Input: part model. Units: mm. Frame: model coordinates. A direction names the side the tool comes from. Round coordinates to 2 decimals unless told otherwise and drop trailing zeros. Write each loop counter-clockwise with the first axis right and the second up, starting at its lowest first coordinate (ties: lowest second). Pieces come first, ordered by that corner, then holes. Notation, with made-up numbers: (40.25, 44.25) - (46.25, 44.25) arc R6 ccw to (46.25, 52.25) - close; hole circle Ø7 at (66, 40.5). An arc over 180 degrees is marked (long way). Use one line per item in the form item = value.
```python
from build123d import *

# Parameters (mm, degrees)
F0_R     = 30.5
F1_DEPTH = 12
F0_R_2   = 5.5
F2_DEPTH = 3


with BuildPart() as f1:
    # F0 (on Top) → F1 (new body)
    with BuildSketch(Plane.XY):
        with Locations((-0.117735, 0.149164)):
            Circle(F0_R)
        with BuildLine():
            ThreePointArc((-18.165188, 22.593082), (-17.375002, 23.206196), (-16.564005, 23.791503))
            ThreePointArc((-16.564005, 23.791503), (22.939297, 17.406431), (17.929717, -22.294755))
            ThreePointArc((17.929717, -22.294755), (17.139532, -22.907869), (16.328534, -23.493176))
            ThreePointArc((16.328534, -23.493176), (-23.174768, -17.108103), (-18.165188, 22.593082))
        make_face(mode=Mode.SUBTRACT)
    extrude(amount=F1_DEPTH)

    # F0 (on Top) → F2 (join)
    with BuildSketch(Plane.XY):
        with BuildLine():
            Line((-3.165644, 5.890266), (-16.564005, 23.791503))
            ThreePointArc((-16.564005, 23.791503), (-17.375002, 23.206196), (-18.165188, 22.593082))
            Line((-18.165188, 22.593082), (-4.766827, 4.691844))
            ThreePointArc((-4.766827, 4.691844), (-5.321579, -3.745706), (2.930173, -5.591938))
            Line((2.930173, -5.591938), (16.328534, -23.493176))
            ThreePointArc((16.328534, -23.493176), (17.139532, -22.907869), (17.929717, -22.294755))
            Line((17.929717, -22.294755), (4.531356, -4.393517))
            ThreePointArc((4.531356, -4.393517), (5.086109, 4.044033), (-3.165644, 5.890266))
        make_face()
        with Locations((-0.117735, 0.149164)):
            Circle(F0_R_2, mode=Mode.SUBTRACT)
    extrude(amount=F2_DEPTH)


solid = f1.part
```
(1) Cut plane C-C on x = 22. Output: boundary loops of the cut face in (y, z).
Derived:
outline = (-20.85, 0) - (-18.3, 0) - (-18.3, 12) - (-20.85, 12) - close; (18.59, 0) - (21.15, 0) - (21.15, 12) - (18.59, 12) - close
(2) Draft query along X for faces 1 (the face through (5.16, 3.94, 1.48)), 2 (the face through (16.279, 25.867, 5.916)), 3 (the face through (9.54, -14.42, 1.48)), 4 (the face through (11, -27, 12)). Return one class per face: released by +X, released by -X, zero draft, split by the parting line, or undercut.
Derived:
face_1 = undercut
face_2 = split by the parting line
face_3 = undercut
face_4 = zero draft
(3) First-contact query: pin 1 Ø4 at (y, z) = (19, 10.5) entering from -X; pin 2 Ø1.5 at (y, z) = (-9, 2) entering from -X; pin 3 Ø5 at (x, z) = (1.5, 1.5) entering from +Y. Flat tips, straight axial feed; report the tip coordinate or a pass-through.
Derived:
pin_1 = -25.54
pin_2 = -29.44
pin_3 = 30.65
(4) Cut plane A-A on x = -8. Output: boundary loops of the cut face in (y, z).
Derived:
outline = (-29.31, 0) - (-27.55, 0) - (-27.55, 12) - (-29.31, 12) - close; (9.01, 0) - (12.35, 0) - (12.35, 3) - (9.01, 3) - close; (27.85, 0) - (29.61, 0) - (29.61, 12) - (27.85, 12) - close
(5) Material intervals for L1, parallel to Y at x = 14, z = 1.5; L2, parallel to X at y = -13, z = 1.75; L3, parallel to X at y = -10, z = 2.75, sorted ascending.
Derived:
L1 = -26.89 to -24.95, -20.38 to -17.04, 25.25 to 27.19
L2 = -27.64 to -25.74, 8.47 to 10.97, 25.51 to 27.4
L3 = -28.88 to -27.07, 6.23 to 8.73, 26.83 to 28.64
(6) Access query for faces 5 (the face through (-11.56, 13.77, 1.48)), 6 (the face through (1, 6, 3)), 7 (the face through (4, -4, 0)). Directions: +Z, -Z, +X, -X, +Y, -Y. A direction counts if a zero-diameter tool reaches every point of the face in a straight line with its end or side. Return the directions, or none.
Derived:
face_5 = +Z, -Z
face_6 = +Z
face_7 = -Z, +X, -X, +Y, -Y
(7) Cut plane B-B on y = -20.5. Output: boundary loops of the cut face in (x, z), then the cut area to 3 significant figures.
Derived:
outline = (-22.56, 0) - (-20.19, 0) - (-20.19, 12) - (-22.56, 12) - close; (14.09, 0) - (16.59, 0) - (16.59, 3) - (14.09, 3) - close; (19.96, 0) - (22.33, 0) - (22.33, 12) - (19.96, 12) - close
area = 64.4 mm^2
